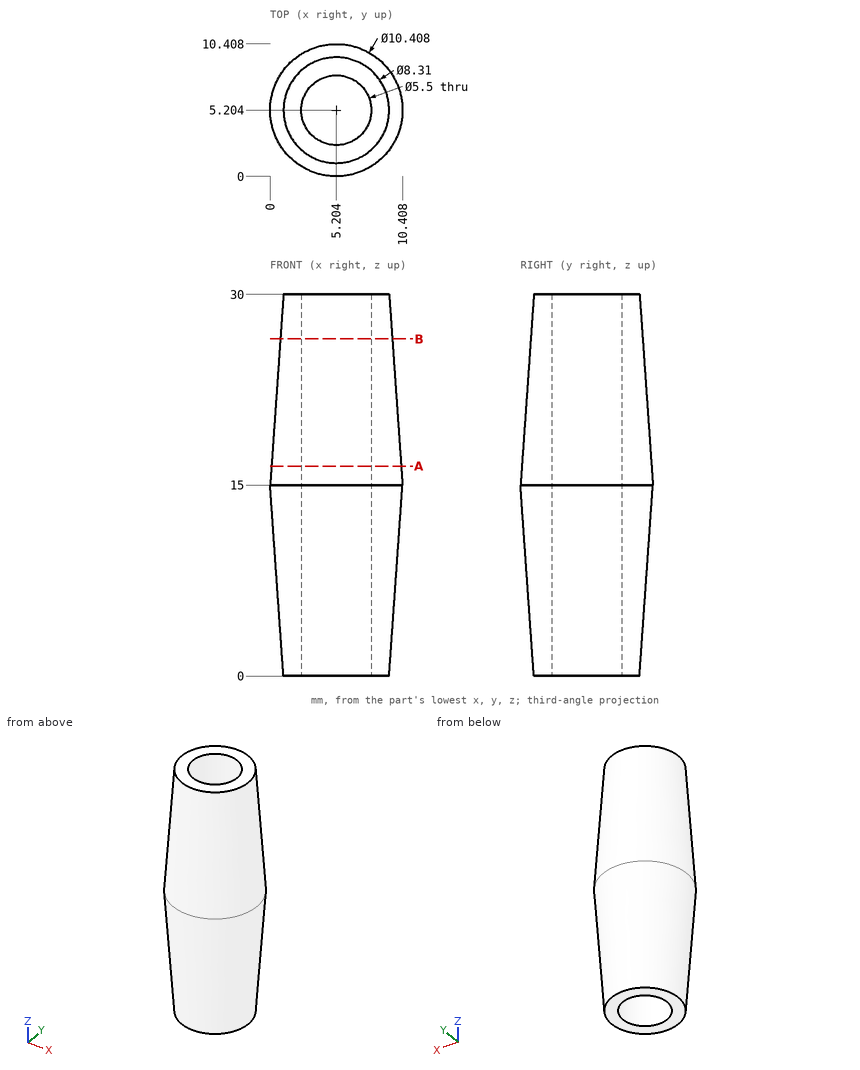
Job drawing, mm, ordinate dimensions from the low corner. One solid piece. Round coordinates to 2 decimals unless told otherwise and drop trailing zeros. Loops run counter-clockwise (first coordinate to the right, second up) from the corner with the lowest first, then second, coordinate; pieces in that order, holes last. Notation, with made-up numbers: (-33.5, -19) -> (16.5, -19) arc R19 ccw to (16.5, 0) -> close; hole circle Ø8 at (-7.75, 37). An arc over 180 degrees is marked (long way). Use CSV: the item, a comma, the result in double quotes. Start each with the question number.
Q1. Drill centre lines: L1, parallel to X at y = 6.75, z = 4.5; L2, parallel to X at y = 2.75, z = 6.5 (1 decimal); L3, parallel to X at y = 8.5, z = 16.5 (1 decimal). Where is each one in solid material? Low to high.
Q2. Flat gauge pins, fed straight in: pin 1 Ø5 at (y, z) = (6, 19.5) entering from +X; pin 2 Ø5 at (x, y) = (5.2, 5.2) entering from +Z; pin 3 Ø6 at (y, z) = (8, 19) entering from +X; pin 4 Ø5 at (y, z) = (4, 8.5) entering from +X. Where does each tip first touch, or does it go through?
Q3. Saw through at A-A on z = 16.5. Give the cut face in (x, y), and give its area (3 significant figures).
Q4. Saw through at B-B on z = 26.5. Give the cut face in (x, y).
Solutions:
1,L1,"x = 1.01 to 2.93, 7.48 to 9.4"
1,L2,"x = 1.3 to 4, 6.4 to 9.1"
1,L3,"x = 1.3 to 9.1"
2,pin 1,"stops at x = 10.26"
2,pin 2,"passes through"
2,pin 3,"stops at x = 10.24"
2,pin 4,"stops at x = 10.11"
3,outline,"circle Ø10.2 at (5.2, 5.2); hole circle Ø5.5 at (5.2, 5.2)"
3,area,"57.9 mm^2"
4,outline,"circle Ø8.8 at (5.2, 5.2); hole circle Ø5.5 at (5.2, 5.2)"
